Geometry: see drawing. Coordinates: mm, zero at the bounding-box minimum. Round coordinates to 2 decimals unless told otherwise and drop trailing zeros. Write each loop counter-clockwise with the first axis right and the second up, starting at its lowest first coordinate (ties: lowest second). Pieces come first, ordered by that corner, then holes. Notation, with made-up numbers: M 67,51.25 L 94,51.25 A24 cw 94,89.25 Z; hole C -9,27 d6. An arc over 180 degrees is marked long. Use one line per item in the form item = value. Start each with the question number.
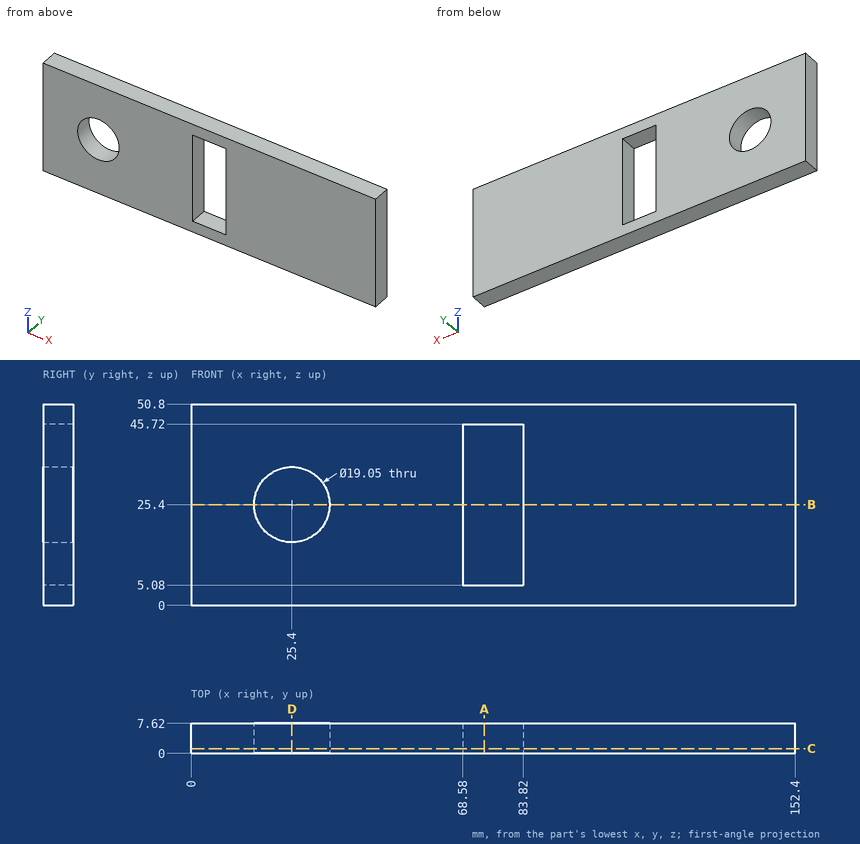
Item 1: First-contact query: pin 1 (11.5 mm diameter, centred on x = 25.4, z = 25.4, fed in from +Y). Flat tip, straight axial feed; report the tip coordinate or a pass-through.
Item 2: Cut plane C-C (y = 1.25). Output: boundary loops of the cut face in (x, z) (3 decimals), plus the area to 3 significant figures.
Item 3: Cut plane B-B (z = 25.4). Output: boundary loops of the cut face in (x, y) (3 decimals), plus the area to 3 significant figures.
Item 4: Cut plane A-A (x = 74). Output: boundary loops of the cut face in (y, z).
Item 5: Cut plane D-D (x = 25.4). Output: boundary loops of the cut face in (y, z) (3 decimals).
Item 6: Ray query, line 1 (X direction, y = 3.25, z = 25.4) (3 decimals); line 2 (X direction, y = 6.25, z = 41); line 3 (X direction, y = 6, z = 17). Return the intervals inside material, ascending. Write a range as from..to.
Final values:
q1.pin_1 = through
q2.outline = M 0,0 L 152.4,0 L 152.4,50.8 L 0,50.8 Z; hole C 25.4,25.4 d19.05; hole M 68.58,5.08 L 83.82,5.08 L 83.82,45.72 L 68.58,45.72 Z
q2.area = 6,840 mm^2
q3.outline = M 0,0 L 15.875,0 L 15.875,7.62 L 0,7.62 Z; M 34.925,0 L 68.58,0 L 68.58,7.62 L 34.925,7.62 Z; M 83.82,0 L 152.4,0 L 152.4,7.62 L 83.82,7.62 Z
q3.area = 900 mm^2
q4.outline = M 0,0 L 7.62,0 L 7.62,5.08 L 0,5.08 Z; M 0,45.72 L 7.62,45.72 L 7.62,50.8 L 0,50.8 Z
q5.outline = M 0,0 L 7.62,0 L 7.62,15.875 L 0,15.875 Z; M 0,34.925 L 7.62,34.925 L 7.62,50.8 L 0,50.8 Z
q6.line_1 = 0..15.875, 34.925..68.58, 83.82..152.4
q6.line_2 = 0..68.58, 83.82..152.4
q6.line_3 = 0..20.91, 29.89..68.58, 83.82..152.4
